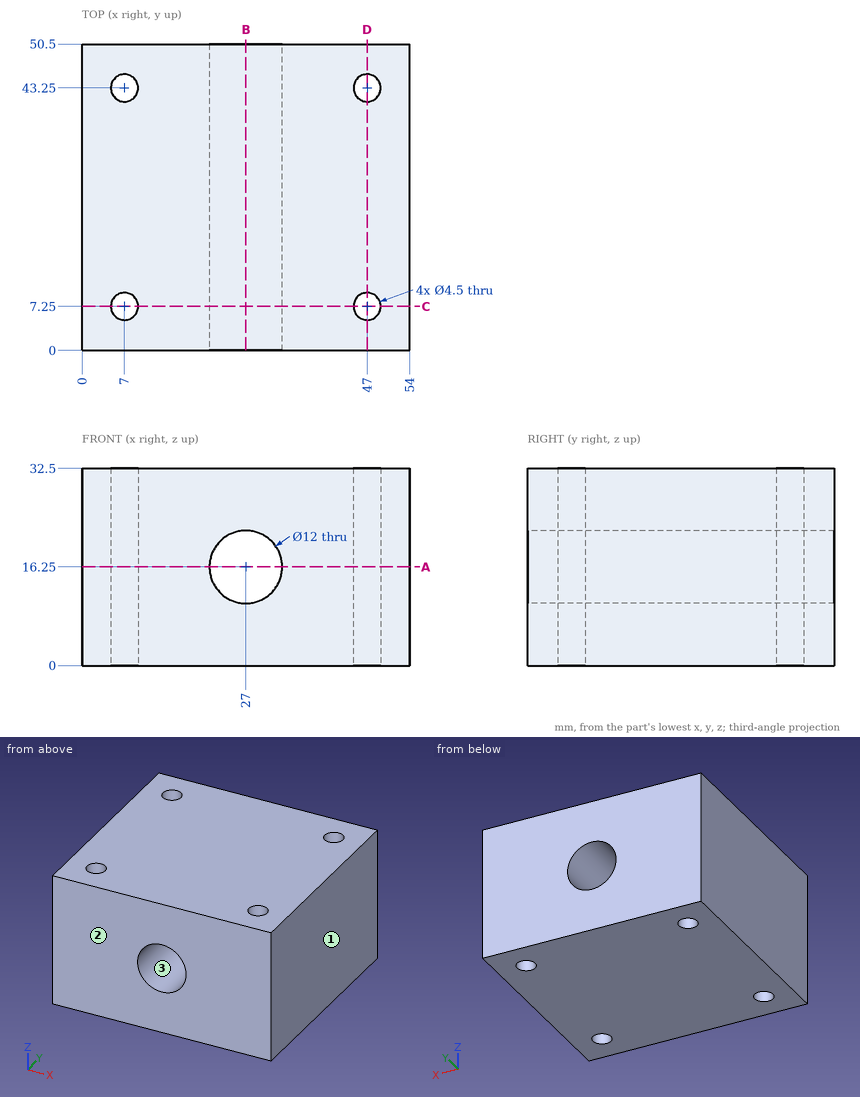
Job drawing, mm, ordinate dimensions from the low corner. One solid piece. Round coordinates to 2 decimals unless told otherwise and drop trailing zeros. Loops run counter-clockwise (first coordinate to the right, second up) from the corner with the lowest first, then second, coordinate; pieces in that order, holes last.
Item 1: Cut at C-C, the plane y = 7.25. Give the cut face in (x, z).
Item 2: Drill centre lines: line 1 (Y direction, x = 47, z = 9); line 2 (X direction, y = 43, z = 14); line 3 (X direction, y = 43, z = 18). Where is each one in solid material? Low to high.
Item 3: Mould opens along X. For the marked faces 1, 2 and 3 say: +X half, -X half, draft (parallel to the pull), parting line (faces both ways), or undercut.
Item 4: Cut at B-B, the plane x = 27. Give the cut face in (y, z).
Item 5: Cut at A-A, the plane z = 16.25. Give the cut face in (x, y), then the cut area to 3 significant figures.
Item 6: Cut at D-D, the plane x = 47. Give the cut face in (y, z), then the cut area to 3 significant figures.
A:
1. outline: (0, 0) - (4.75, 0) - (4.75, 32.5) - (0, 32.5) - close; (9.25, 0) - (44.75, 0) - (44.75, 32.5) - (9.25, 32.5) - close; (49.25, 0) - (54, 0) - (54, 32.5) - (49.25, 32.5) - close; hole circle Ø12 at (27, 16.25)
2. line 1: y = 0 to 5, 9.5 to 41, 45.5 to 50.5
2. line 2: x = 0 to 4.76, 9.24 to 21.44, 32.56 to 44.76, 49.24 to 54
2. line 3: x = 0 to 4.76, 9.24 to 21.26, 32.74 to 44.76, 49.24 to 54
3. face 1: +X half
3. face 2: draft
3. face 3: undercut
4. outline: (0, 0) - (50.5, 0) - (50.5, 10.25) - (0, 10.25) - close; (0, 22.25) - (50.5, 22.25) - (50.5, 32.5) - (0, 32.5) - close
5. outline: (0, 0) - (21, 0) - (21, 50.5) - (0, 50.5) - close; (33, 0) - (54, 0) - (54, 50.5) - (33, 50.5) - close; hole circle Ø4.5 at (7, 7.25); hole circle Ø4.5 at (7, 43.25); hole circle Ø4.5 at (47, 7.25); hole circle Ø4.5 at (47, 43.25)
5. area: 2,060 mm2
6. outline: (0, 0) - (5, 0) - (5, 32.5) - (0, 32.5) - close; (9.5, 0) - (41, 0) - (41, 32.5) - (9.5, 32.5) - close; (45.5, 0) - (50.5, 0) - (50.5, 32.5) - (45.5, 32.5) - close
6. area: 1,350 mm2
